from build123d import *

# Parameters (mm, degrees)
F1_DEPTH  = 15.24
F2_W      = 22.628388
F2_H      = 18.998165
F3_DEPTH  = 14.0208
F5_DEPTH  = 23.622
F6_DEPTH  = 0.8636
F7_R      = 3.766299
F7_R_2    = 2.625981
F8_DEPTH  = 0.6604
F9_R      = 2.413
F10_DEPTH = 11.938


with BuildPart() as f1:
    # F0 (on Front) → F1 (new body)
    with BuildSketch(Plane.XZ):
        Polygon((3.550537, 0), (0, 0), (0, -10.214623), (25.4, -10.214623), (25.4, 0), (21.685589, 0), (20.48387, -5.08), (5.844731, -5.08), align=None)
    extrude(amount=F1_DEPTH)

    # F2 (on Front) → F3 (join)
    with BuildSketch(Plane.XZ):
        with Locations((12.809009, 3.497728)):
            Rectangle(F2_W, F2_H)
    extrude(amount=F3_DEPTH)

    # F4 (on face) → F5 (join)
    with BuildSketch(Plane.YZ.offset(24.123203)):
        Polygon((-7.100273, 9.703922), (-9.255558, 8.901955), (-10.212499, 6.810862), (-9.410532, 4.655577), (-7.319439, 3.698636), (-5.164154, 4.500603), (-4.207213, 6.591696), (-5.00918, 8.746981), align=None)
    extrude(amount=-F5_DEPTH)

    # F4 (on face) → F6 (join)
    with BuildSketch(Plane.YZ.offset(24.123203)):
        Polygon((-7.100273, 9.703922), (-9.255558, 8.901955), (-10.212499, 6.810862), (-9.410532, 4.655577), (-7.319439, 3.698636), (-5.164154, 4.500603), (-4.207213, 6.591696), (-5.00918, 8.746981), align=None)
    extrude(amount=F6_DEPTH)

    # F7 (on face) → F8 (join)
    with BuildSketch(Plane.XZ.offset(14.0208)):
        with Locations((7.834505, 6.848152)):
            Circle(F7_R)
        with Locations((18.51875, 6.644643)):
            Circle(F7_R_2)
    extrude(amount=F8_DEPTH)

    # F9 (on face) → F10 (join)
    with BuildSketch(Plane(origin=(0, 0, -10.214623), x_dir=(1, 0, 0), z_dir=(0, 0, -1))):
        with Locations((12.7, 7.62)):
            Circle(F9_R)
    extrude(amount=F10_DEPTH)


solid = f1.part
Work out the finished part from the listing and answer in its coordinate system (mm). A direction names the side the tool comes from. Give positions to 0.01 mm unless a question says otherwise; leave off trailing zeros. Write each loop counter-clockwise with the first axis right and the second up, starting at its lowest first coordinate (ties: lowest second). Pieces come first, ordered by that corner, then holes. Notation, with made-up numbers: (-3, 36) - (40, 36) arc R26 cw to (40, 66) - close; hole circle Ø1 at (-20, -6.5). An arc over 180 degrees is marked (long way). One line per item, written item: value. Start each with the question number.
1. Consider probe 1 along Z at (x, y) = (11, -12.25); probe 2 along Y at (x, z) = (14.25, 0); probe 3 along X at (y, z) = (-8.25, 9.5). Determine where each line is inside the solid, lowest interval first.
2. For a pull along Z with two mould halves and no side action, classify faces 1 (the flat face through (13, 0, 2)), 2 (the flat face through (24.123, -4, 7)), 3 (the flat face through (1, -9.73, 7.87)) as +Z half, -Z half, draft (parallel to the pull), parting line (faces both ways), or undercut.
3. Find section A-A (x = 3). Write down the section's boundary in (y, z), then the cut area to 3 significant figures.
4. For faces 4 (the flat face through (1, -4.6, 7.65)), 5 (the flat face through (4.714, -14.622, -2.576)), 6 (the flat face through (24.549, -6.257, 4.094)), 7 (the flat face through (24.55, -4.6, 7.65)), 8 (the flat face through (18, -14.681, 7)), determine the directions among +Z, -Z, +X, -X, +Y, -Y from which every point of the face is accessible in a straight line to the end or side of a thin tool.
5. Find section D-D (x = 12.7). Write down the section's boundary in (y, z).
6. Find section C-C (z = -16). Write down the section's boundary in (x, y), then the cut area to 3 significant figures.
7. Given pin 1 (6 mm diameter, centred on x = 18.5, z = 6.5, fed in from -Y); pin 2 (1.5 mm diameter, centred on x = 10, y = -10, fed in from -Z); pin 3 (5 mm diameter, centred on y = -8.5, z = 5.5, fed in from +X), each flat-ended and moving along its own axis, determine where each tip first touches the part or whether it passes through.
8. Find section B-B (y = -1). Write down the section's boundary in (x, z).
Geometry results:
1. probe 1: -10.21 to 13
1. probe 2: -14.02 to 0
1. probe 3: 1.49 to 24.12
2. face 1: draft
2. face 2: undercut
2. face 3: +Z half
3. outline: (-15.24, -10.21) - (0, -10.21) - (0, 13) - (-14.02, 13) - (-14.02, 0) - (-15.24, 0) - close
3. area: 338 mm2
4. face 4: +Z, -X, +Y
4. face 5: -Y
4. face 6: +X, +Y
4. face 7: +Z, +X, +Y
4. face 8: +Z, +X, -X, -Y
5. outline: (-15.24, -10.21) - (-10.03, -10.21) - (-10.03, -22.15) - (-5.21, -22.15) - (-5.21, -10.21) - (0, -10.21) - (0, 13) - (-14.02, 13) - (-14.02, -5.08) - (-15.24, -5.08) - close
6. outline: circle Ø4.83 at (12.7, -7.62)
6. area: 18.3 mm2
7. pin 1: y = -14.68
7. pin 2: z = -10.21
7. pin 3: x = 24.99
8. outline: (0, -10.21) - (25.4, -10.21) - (25.4, 0) - (24.12, 0) - (24.12, 13) - (1.49, 13) - (1.49, 0) - (0, 0) - close
